Model file for the job. Use its own axes, mm. Face numbers are marked on the shaded views. A direction names the side the tool comes from. Give positions to 0.01 mm unless a question says otherwise; leave off trailing zeros. Write each loop counter-clockwise with the first axis right and the second up, starting at its lowest first coordinate (ties: lowest second). Pieces come first, ordered by that corner, then holes.
```python
from build123d import *

# Parameters (mm, degrees)
F1_DEPTH    = 33
F3_DEPTH    = 21.001
F4_DEPTH    = 3
F6_T1_DEPTH = 35.508521627
F6_T3_DEPTH = 36.4826554363
F7_W        = 21
F7_H        = 2
F8_DEPTH    = 10
F9_W        = 21
F9_H        = 1
F10_DEPTH   = 1
F11_SIZE2   = 0.8660254038
F11_SIZE    = 0.5
F12_R       = 0.99999


# Not quite as in the source:
# - a fillet or chamfer that OpenCascade refuses, or shapes differently, is made with other operations: its cross-section is extruded or revolved along the edge and cut away or added
# - a fillet or chamfer is up to 0.001 mm smaller than in the source, because OpenCascade refuses the exact size
# - a pattern or mirror of a feature is missing from the dataset's text; its kind, count and spacing are read off the source's solid


with BuildPart() as f1:
    # F0 (on Top) → F1 (new body)
    with BuildSketch(Plane.XY):
        Polygon((-33.9465141296, 18.5), (-33.9465141296, 15), (-26.4407399079, 15), align=None)
        Polygon((-20.4522883514, 15), (-12.9465141296, 15), (-12.9465141296, 18.5), align=None)
        with BuildLine():
            Line((-33.9465141296, 15), (-33.9465141296, 0))
            ThreePointArc((-33.9465141296, 0), (-23.4465141296, 1.783504535), (-12.9465141296, 0))
            Line((-12.9465141296, 0), (-12.9465141296, 15))
            Line((-12.9465141296, 15), (-20.4522883514, 15))
            Line((-20.4522883514, 15), (-26.4407399079, 15))
            Line((-26.4407399079, 15), (-33.9465141296, 15))
        make_face()
    extrude(amount=F1_DEPTH)

    # F2 (on face) → F3 (cut, through all)
    with BuildSketch(Plane.YZ.offset(-12.9465141296)):
        Polygon((18.5, 0), (18.5, 33), (17.75, 0), align=None)
    extrude(amount=-F3_DEPTH, mode=Mode.SUBTRACT)

    # F2 (on face) → F4 (cut)
    with BuildSketch(Plane.YZ.offset(-12.9465141296)):
        Polygon((15.25, 0), (16.5, 33), (13.5, 33), (13.25, 0), align=None)
    f4 = extrude(amount=-F4_DEPTH, mode=Mode.SUBTRACT)

    # F4_copies: F4 across plane
    add(f4.mirror(Plane(origin=(-23.446514, 0, 0), x_dir=(0, 0, -1), z_dir=(-1, 0, 0))), mode=Mode.SUBTRACT)

    # F6: fillet of radius 0.5 on 4 edges, made by hand

    # F6_s2 → F6_t1 (cut)
    with BuildSketch(Plane(origin=(0, 0.7875654118, 34.6528781205), x_dir=(1, 0, 0), z_dir=(0, -0.0227214054, -0.9997418355))):
        with BuildLine():
            add(Edge.make_bspline(
                [(-13.4465141296, -17.7454175809), (-12.9465141296, -17.7454175809), (-12.9465141296, -17.2454175809)],
                knots=[0, 0, 0, 1, 1, 1], degree=2, weights=[1, 1, 1]))
            Line((-12.9465141296, -17.2454175809), (-12.9465141296, -17.7454175809))
            Line((-12.9465141296, -17.7454175809), (-13.4465141296, -17.7454175809))
        make_face()
        with BuildLine():
            add(Edge.make_bspline(
                [(-33.9465141296, -17.2454175809), (-33.9465141296, -17.7454175809), (-33.4465141296, -17.7454175809)],
                knots=[0, 0, 0, 1, 1, 1], degree=2, weights=[1, 1, 1]))
            Line((-33.4465141296, -17.7454175809), (-33.9465141296, -17.7454175809))
            Line((-33.9465141296, -17.7454175809), (-33.9465141296, -17.2454175809))
        make_face()
    extrude(amount=F6_T1_DEPTH, mode=Mode.SUBTRACT)

    # F6_s4 → F6_t3 (cut)
    with BuildSketch(Plane.XY.offset(-1.7413277182)):
        with BuildLine():
            add(Edge.make_bspline(
                [(-33.291715368, 0.2210972397), (-33.9465141296, 0.0078982049), (-33.9465141296, 0.6965310873)],
                knots=[0, 0, 0, 1, 1, 1], degree=2, weights=[1, 1, 1]))
            Line((-33.9465141296, 0.6965310873), (-33.9465141296, 0))
            ThreePointArc((-33.9465141296, 0), (-33.6197154132, 0.1123275396), (-33.291715368, 0.2210972397))
        make_face()
        with BuildLine():
            add(Edge.make_bspline(
                [(-12.9465141296, 0.6965310873), (-12.9465141296, 0.0078982049), (-13.6013128912, 0.2210972397)],
                knots=[0, 0, 0, 1, 1, 1], degree=2, weights=[1, 1, 1]))
            ThreePointArc((-13.6013128912, 0.2210972397), (-13.2733128461, 0.1123275396), (-12.9465141296, 0))
            Line((-12.9465141296, 0), (-12.9465141296, 0.6965310873))
        make_face()
    extrude(amount=F6_T3_DEPTH, mode=Mode.SUBTRACT)

    # F7 (on face) → F8 (join)
    with BuildSketch(Plane(origin=(0, 0, 0), x_dir=(1, 0, 0), z_dir=(0, 0, -1))):
        with Locations((-23.4465141296, -12.25)):
            Rectangle(F7_W, F7_H)
    extrude(amount=F8_DEPTH)

    # F9 (on face) → F10 (join)
    with BuildSketch(Plane(origin=(0, 13.25, 0), x_dir=(-1, 0, 0), z_dir=(0, 1, 0))):
        with Locations((23.4465141296, -2.5)):
            Rectangle(F9_W, F9_H)
    extrude(amount=F10_DEPTH)

    # F11
    f11_edges = [f1.edges().sort_by_distance(p)[0] for p in [
        (-23.446514, 14.25, -2),
    ]]
    f11_side = f1.faces().sort_by_distance((-23.446514, 13.75, -2))[0]
    chamfer(f11_edges, length=F11_SIZE, length2=F11_SIZE2, reference=f11_side)

    # F12 (radius 1 in the source; OpenCascade refuses exactly that, so slightly less here)
    f12_edges = [f1.edges().sort_by_distance(p)[0] for p in [
        (-23.446514, 11.25, 0),
        (-23.446514, 13.25, -10),
        (-23.446514, 11.25, -10),
    ]]
    fillet(f12_edges, radius=F12_R)


solid = f1.part
```
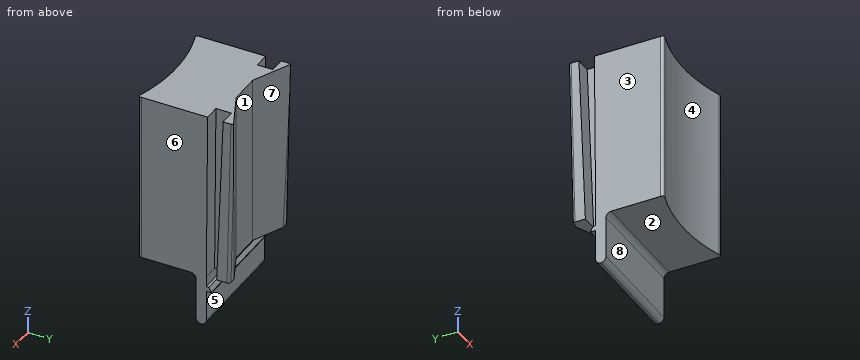
1. Slice it at A-A, the plane y = 15.75. Write the cut outline in (x, z).
Calculated:
outline: (-33.95, 0) - (-28.05, 0) - (-28.05, 33) - (-30.95, 33) - (-30.95, 13.2) - (-33.95, 13.2) - close; (-18.84, 0) - (-12.95, 0) - (-12.95, 13.2) - (-15.95, 13.2) - (-15.95, 33) - (-18.84, 33) - close
2. Pull direction X, two halves, no side cores. Call the marked faces 1, 2, 3 and 4: +X half, -X half, draft (parallel to the pull), parting line (faces both ways), or undercut.
Calculated:
face 1: undercut
face 2: draft
face 3: -X half
face 4: undercut
3. Which spindle directions (+Z, -Z, +X, -X, +Y, -Y) get a long thin tool onto all of the face, cutting with end or side? Do the marked faces 5, 6, 7 and 8. Say none if no direction does.
Calculated:
face 5: -Z, +X, -X, +Y
face 6: +Z, -Z, +X, +Y, -Y
face 7: +Z, -Z, +Y
face 8: -Z, +X, -X, -Y
4. Slice it at C-C, the plane z = -6.5. Write the cut outline in (x, y).
Calculated:
outline: (-33.95, 11.25) - (-12.95, 11.25) - (-12.95, 13.25) - (-33.95, 13.25) - close
5. Pin check, flat tips, straight feed: P1, Ø6, axis at x = -16, y = 16, coming from the -Z side; P2, Ø3, axis at x = -27.5, z = -5.5, coming from the +Y side; P3, Ø1, axis at x = -24.5, y = 14, coming from the -Z side. Stop position of each tip, or through.
Calculated:
P1: stops at z = -9.66
P2: stops at y = 13.25
P3: stops at z = -3
6. Probe probe 1 along Z at (x, y) = (-27.5, 5.25); probe 2 along X at (y, z) = (14.25, 22); probe 3 along Y at (x, z) = (-24, 0.5). List the from-to ranges inside material, lowest first.
Calculated:
probe 1: z = 0 to 33
probe 2: x = -30.95 to -15.95
probe 3: y = 1.78 to 15
7. Slice it at D-D, the plane y = 3. Write the cut outline in (x, z), and give its area (3 significant figures).
Calculated:
outline: (-33.95, 0) - (-12.95, 0) - (-12.95, 33) - (-33.95, 33) - close
area: 693 mm2
